```python
from build123d import *

# Parameters (mm, degrees)
SKETCH1_W                 = 5.2
SKETCH1_H                 = 14
SKETCH1_R                 = 3.2
SKETCH1_R_2               = 1.7
SKETCH1_R_3               = 2.75
BOSS_EXTRUDE1_DEPTH       = 10
SKETCH2_R                 = 2.6
CUT_EXTRUDE1_DEPTH        = 20
SKETCH3_R                 = 5.1
CUT_EXTRUDE2_DEPTH        = 15.2
BOSS_EXTRUDE2_DEPTH       = 0.45
BOSS_EXTRUDE2_DEPTH_BACK  = 0.45
SKETCH4_R                 = 5.1
SKETCH4_R_2               = 4.7
BOSS_EXTRUDE3_DEPTH       = 0.45
BOSS_EXTRUDE3_DEPTH_BACK  = 0.45
SKETCH5_R                 = 5.1
SKETCH5_R_2               = 4.7
CUT_EXTRUDE3_START        = -11
CUT_EXTRUDE3_OUTLINE_W    = 2.009975124
CUT_EXTRUDE3_OUTLINE_H    = 0.9
CUT_EXTRUDE3_OUTLINE_W_2  = 3
CUT_EXTRUDE3_OUTLINE_H_2  = 19.2
CUT_EXTRUDE3_DEPTH        = 12
SKETCH7_R                 = 12.5
CUT_EXTRUDE4_DEPTH        = 1
SKETCH8_R                 = 9.6
CUT_EXTRUDE5_DEPTH        = 1
SKETCH11_R                = 17
CUT_EXTRUDE6_DEPTH        = 6
BOSS_EXTRUDE4_OUTLINE_W   = 7.810507711
BOSS_EXTRUDE4_OUTLINE_H   = 8
BOSS_EXTRUDE4_OUTLINE_W_2 = 8
BOSS_EXTRUDE4_DEPTH       = 4.5
SKETCH13_R                = 2.125
CUT_EXTRUDE7_DEPTH        = 9.5
SKETCH16_W                = 0.189492289
SKETCH16_H                = 3.060913179
CUT_EXTRUDE8_DEPTH        = 4.5
FILLET1_R                 = 8
SKETCH19_R                = 12.5
CUT_EXTRUDE9_DEPTH        = 5
FILLET3_R                 = 3
CUT_EXTRUDE10_REACH       = 116.689
SKETCH20_R                = 1.7


with BuildPart() as part:
    # Sketch1 → Boss-Extrude1 (new body)
    with BuildSketch(Plane(origin=(0, 0, 0), x_dir=(0, 1, 0), z_dir=(0, 0, 1))):
        with BuildLine():
            Line((44.859200041, 91.5), (44.859200041, 77.3))
            Line((44.859200041, 77.3), (39.859200041, 77.3))
            Line((39.859200041, 77.3), (12.058048672, 27.485891377))
            ThreePointArc((12.058048672, 27.485891377), (12.182830244, 16.059150365), (22.1, 10.381499035))
            Line((22.1, 10.381499035), (33.6, 10.381499035))
            ThreePointArc((33.6, 10.381499035), (36.198905176, 18.091500699), (40.42011322, 25.047062246))
            Line((40.42011322, 25.047062246), (40.42011322, 39.489492289))
            Line((40.42011322, 39.489492289), (82.859200041, 39.489492289))
            Line((82.859200041, 39.489492289), (82.859200041, 77.3))
            Line((82.859200041, 77.3), (64.059200041, 77.3))
            Line((64.059200041, 77.3), (64.059200041, 91.5))
            Line((64.059200041, 91.5), (44.859200041, 91.5))
        make_face()
        with Locations((78.259200041, 52.489492289)):
            Rectangle(SKETCH1_W, SKETCH1_H, mode=Mode.SUBTRACT)
        with Locations(Location((22.1, 21.881499035, 0), (0, 0, 270))):
            Circle(SKETCH1_R, mode=Mode.SUBTRACT)
        with Locations(Location((65.859200041, 58.3, 0), (0, 0, 270))):
            Circle(SKETCH1_R_2, mode=Mode.SUBTRACT)
        with Locations(Location((56.359200041, 48.8, 0), (0, 0, 270))):
            Circle(SKETCH1_R_2, mode=Mode.SUBTRACT)
        with Locations(Location((46.859200041, 58.3, 0), (0, 0, 270))):
            Circle(SKETCH1_R_2, mode=Mode.SUBTRACT)
        with Locations(Location((56.359200041, 58.3, 0), (0, 0, 270))):
            Circle(SKETCH1_R_3, mode=Mode.SUBTRACT)
        with Locations(Location((56.359200041, 67.8, 0), (0, 0, 270))):
            Circle(SKETCH1_R_2, mode=Mode.SUBTRACT)
    extrude(amount=BOSS_EXTRUDE1_DEPTH)

    # Sketch2 → Cut-Extrude1 (cut)
    with BuildSketch(Plane.XZ.offset(-44.859200041)):
        with Locations(Location((-82.4, 5, 0), (0, 0, 270))):
            Circle(SKETCH2_R)
    extrude(amount=-CUT_EXTRUDE1_DEPTH, mode=Mode.SUBTRACT)

    # Sketch3 → Cut-Extrude2 (cut)
    with BuildSketch(Plane(origin=(0, 46.859200041, 0), x_dir=(-1, 0, 0), z_dir=(0, -1, 0))):
        with Locations((82.4, -5)):
            Circle(SKETCH3_R)
    extrude(amount=-CUT_EXTRUDE2_DEPTH, mode=Mode.SUBTRACT)

    # Sketch4 → Boss-Extrude2 (add, two sides: drawn at the far end of the back side and taken through both)
    with BuildSketch(Plane(origin=(0, 51.909200041, 0), x_dir=(-1, 0, 0), z_dir=(0, -1, 0)).offset(-BOSS_EXTRUDE2_DEPTH_BACK)):
        with Locations((82.4, -5)):
            Circle(SKETCH4_R)
        with Locations(Location((82.4, -5, 0), (0, 0, 90))):
            Circle(SKETCH4_R_2, mode=Mode.SUBTRACT)
    extrude(amount=BOSS_EXTRUDE2_DEPTH + BOSS_EXTRUDE2_DEPTH_BACK)

    # Sketch5 → Boss-Extrude3 (add, two sides: drawn at the far end of the back side and taken through both)
    with BuildSketch(Plane(origin=(0, 59.009200041, 0), x_dir=(1, 0, 0), z_dir=(0, 1, 0)).offset(-BOSS_EXTRUDE3_DEPTH_BACK)):
        with Locations((-82.4, -5)):
            Circle(SKETCH5_R)
        with Locations(Location((-82.4, -5, 0), (0, 0, 90))):
            Circle(SKETCH5_R_2, mode=Mode.SUBTRACT)
    extrude(amount=BOSS_EXTRUDE3_DEPTH + BOSS_EXTRUDE3_DEPTH_BACK)

    # Cut-Extrude3: read off the stored shape, not the designer's step
    # Cut-Extrude3 outline → Cut-Extrude3 (cut)
    with BuildSketch(Plane.XY.offset(10).offset(CUT_EXTRUDE3_START)):
        with Locations((-82.4, 59.009200041)):
            Rectangle(CUT_EXTRUDE3_OUTLINE_W, CUT_EXTRUDE3_OUTLINE_H)
        with Locations((-82.4, 51.909200041)):
            Rectangle(CUT_EXTRUDE3_OUTLINE_W, CUT_EXTRUDE3_OUTLINE_H)
        with Locations((-90, 54.459200041)):
            Rectangle(CUT_EXTRUDE3_OUTLINE_W_2, CUT_EXTRUDE3_OUTLINE_H_2)
    extrude(amount=CUT_EXTRUDE3_DEPTH, mode=Mode.SUBTRACT)

    # Sketch7 → Cut-Extrude4 (cut)
    with BuildSketch(Plane.XY.offset(10)):
        with Locations((-21.881499035, 22.1)):
            Circle(SKETCH7_R)
    extrude(amount=-CUT_EXTRUDE4_DEPTH, mode=Mode.SUBTRACT)

    # Sketch8 → Cut-Extrude5 (cut)
    with BuildSketch(Plane.XY.offset(9)):
        with Locations((-21.881499035, 22.1)):
            Circle(SKETCH8_R)
    extrude(amount=-CUT_EXTRUDE5_DEPTH, mode=Mode.SUBTRACT)

    # Sketch11 → Cut-Extrude6 (cut)
    with BuildSketch(Plane.XY.offset(10)):
        with Locations((-58.3, 56.359200041)):
            Circle(SKETCH11_R)
    extrude(amount=-CUT_EXTRUDE6_DEPTH, mode=Mode.SUBTRACT)

    # Boss-Extrude4: read off the stored shape, not the designer's step
    # Boss-Extrude4 outline → Boss-Extrude4 (add)
    with BuildSketch(Plane(origin=(0, 0, 0), x_dir=(1, 0, 0), z_dir=(0, 0, -1))):
        with Locations((-43.394746145, -71.359200041)):
            Rectangle(BOSS_EXTRUDE4_OUTLINE_W, BOSS_EXTRUDE4_OUTLINE_H)
        Polygon((-47.3, -45.359200041), (-39.489492289, -45.359200041), (-39.489492289, -40.42011322), (-39.3, -40.42011322), (-39.3, -37.359200041), (-47.3, -37.359200041), align=None)
        with Locations((-73.3, -71.359200041)):
            Rectangle(BOSS_EXTRUDE4_OUTLINE_W_2, BOSS_EXTRUDE4_OUTLINE_H)
        with Locations((-73.3, -41.359200041)):
            Rectangle(BOSS_EXTRUDE4_OUTLINE_W_2, BOSS_EXTRUDE4_OUTLINE_H)
    extrude(amount=BOSS_EXTRUDE4_DEPTH)

    # Sketch13 → Cut-Extrude7 (cut)
    with BuildSketch(Plane(origin=(0, 0, -4.5), x_dir=(1, 0, 0), z_dir=(0, 0, -1))):
        with Locations(Location((-43.3, -41.359200041, 0), (0, 0, 180))):
            Circle(SKETCH13_R)
        with Locations(Location((-43.3, -71.359200041, 0), (0, 0, 180))):
            Circle(SKETCH13_R)
        with Locations(Location((-73.3, -71.359200041, 0), (0, 0, 180))):
            Circle(SKETCH13_R)
        with Locations(Location((-73.3, -41.359200041, 0), (0, 0, 180))):
            Circle(SKETCH13_R)
    extrude(amount=-CUT_EXTRUDE7_DEPTH, mode=Mode.SUBTRACT)

    # Sketch16 → Cut-Extrude8 (cut)
    with BuildSketch(Plane(origin=(0, 0, -4.5), x_dir=(1, 0, 0), z_dir=(0, 0, -1))):
        with Locations((-39.394746145, -38.88965663)):
            Rectangle(SKETCH16_W, SKETCH16_H)
    extrude(amount=-CUT_EXTRUDE8_DEPTH, mode=Mode.SUBTRACT)

    # Fillet1
    # the kernel refuses this fillet: 8 mm, written as the material it adds along each edge
    with BuildSketch(Plane(origin=(-39.489492289, 40.42011322, 0), x_dir=(0, 1, 0), z_dir=(0, 0, 1))) as fillet1_piece_1:
        with BuildLine():
            CenterArc((FILLET1_R, -FILLET1_R), FILLET1_R, 90, 90)
            Line((0, -FILLET1_R), (0, 0))
            Line((0, 0), (FILLET1_R, 0))
        make_face()
    extrude(amount=10)
    # the kernel refuses this fillet: 8 mm, written as the material it takes off along each edge
    with BuildSketch(Plane(origin=(-25.047062246, 40.42011322, -6.434675881), x_dir=(-1, 0, 0), z_dir=(0, 0, 1))) as fillet1_2_piece_1:
        with BuildLine():
            CenterArc((2.573870352, 8), FILLET1_R, 236.049500449, 33.950499551)
            ThreePointArc((-1.893941258, 1.363836996), (-0.936214399, 0.696855523), (0, 0))
            Line((0, 0), (2.573870352, 0))
        make_face()
    extrude(amount=22.869351762, mode=Mode.SUBTRACT)
    with BuildSketch(Plane(origin=(-10.381499035, 33.6, -14.879687817), x_dir=(-0.9588293573098585, 0.2839828578642794, 0), z_dir=(0, 0, 1))) as fillet1_2_piece_2:
        with BuildLine():
            CenterArc((5.98040435, 7.978695466), FILLET1_R, 196.498058708, 69.319545905)
            Line((-1.690230508, 5.706832603), (0, 0))
            ThreePointArc((0, 0), (2.698475134, 0.098533472), (5.396950267, 0))
        make_face()
    extrude(amount=39.759375634, mode=Mode.SUBTRACT)

    # Sketch19 → Cut-Extrude9 (cut)
    with BuildSketch(Plane.XY.offset(10)):
        with Locations((-21.881499035, 22.1)):
            Circle(SKETCH19_R)
    extrude(amount=-CUT_EXTRUDE9_DEPTH, mode=Mode.SUBTRACT)

    # Fillet3
    # the kernel refuses this fillet: 3 mm, written as the material it takes off along each edge
    with BuildSketch(Plane(origin=(-10.381499035, 26.998979486, 14.214960222), x_dir=(9.684312598090364e-12, 1.0, -1.847411112972132e-14), z_dir=(0, 0, -1))) as fillet3_piece_1:
        with BuildLine():
            CenterArc((3.039490322, 1.812802001), FILLET3_R, 217.17613817, 22.016092035)
            ThreePointArc((1.503012295, -0.763869354), (0.76439954, -0.356565251), (0, 0))
            Line((0, 0), (0.649145388, 0))
        make_face()
    extrude(amount=9.214960222, mode=Mode.SUBTRACT)
    with BuildSketch(Plane(origin=(-31.763744729, 14.445509812, 5), x_dir=(-0.35715309500497466, 0.9340458590071301, -7.501643631045315e-14), z_dir=(0, 0, 1))) as fillet3_piece_2:
        with BuildLine():
            CenterArc((8.109181309, 2.871430927), FILLET3_R, 129.90874339, 123.256431286)
            Line((6.184481226, 5.172632698), (0, 0))
            ThreePointArc((0, 0), (3.620170227, 0.53570447), (7.240340454, 0))
        make_face()
    extrude(amount=25.156254778, mode=Mode.SUBTRACT)

    # Sketch20 → Cut-Extrude10 (cut, up to next)
    with BuildSketch(Plane(origin=(0, 82.859200041, 0), x_dir=(-1, 0, 0), z_dir=(0, 1, 0)), mode=Mode.PRIVATE) as cut_extrude10_sk1:
        with Locations(Location((52.489492289, 5, 0), (0, 0, 90))):
            Circle(SKETCH20_R)
    cut_extrude10_tool1 = extrude(cut_extrude10_sk1.sketch, amount=-CUT_EXTRUDE10_REACH, mode=Mode.PRIVATE) & part.part
    add(cut_extrude10_tool1.solids().sort_by_distance((-52.489492, 82.8592, 5))[0], mode=Mode.SUBTRACT)


solid = part.part
```
CAD build for the part. Positions are in the model's coordinates, mm. A direction names the side the tool comes from. Round coordinates to 2 decimals unless told otherwise and drop trailing zeros. Write each loop counter-clockwise with the first axis right and the second up, starting at its lowest first coordinate (ties: lowest second). Pieces come first, ordered by that corner, then holes. Notation, with made-up numbers: M 31.25,-14.5 L 36.25,-14.5 A19 ccw 36.25,1.5 Z; hole C 7.25,74.25 d1. An arc over 180 degrees is marked long. One line per question, with ' | ' between items.
1. Pin check, flat tips, straight feed: pin 1 Ø5 at (x, z) = (-74, -2) entering from -Y; pin 2 Ø4 at (y, z) = (48.5, 7) entering from +X; pin 3 Ø3.5 at (x, z) = (-44.5, -2.5) entering from -Y. Stop position of each tip, or through.
Working result:
pin 1: y = 37.18 | pin 2: x = -39.26 | pin 3: y = 37.36
2. Cut at A-A on x = -58.3. Write the cut outline in (y, z).
Working result:
outline: M 29.26,0 L 45.16,0 L 45.16,4 L 39.36,4 L 39.36,10 L 29.26,10 Z; M 48.56,0 L 53.61,0 L 53.61,4 L 48.56,4 Z; M 59.11,0 L 64.16,0 L 64.16,4 L 59.11,4 Z; M 67.56,0 L 75.66,0 L 75.66,10 L 73.36,10 L 73.36,4 L 67.56,4 Z; M 80.86,0 L 82.86,0 L 82.86,10 L 80.86,10 Z
3. Mould opens along Z. For faces 1 (the flat face through (-71.6, 73.1, -4.5)), 2 (the cylindrical face through (-71.61, 40.07, 0.18)), 3 (the cylindrical face through (-87.1, 51.9, 5.1)) say: pulls with the +Z half, pulls with the -Z half, needs draft (parallel to the pull), parting line crosses it, or undercut.
Working result:
face 1: pulls with the -Z half | face 2: needs draft | face 3: undercut
4. Probe L1, parallel to Y at x = -73.3, z = -0.5; L2, parallel to X at y = 49, z = 8.75; L3, parallel to X at y = 45.5, z = 5. List the from-to ranges inside material, lowest first. Write a range as from..to.
Working result:
L1: 37.36..39.23, 43.48..45.36, 67.36..69.23, 73.48..75.36 | L2: -88.5..-85.86, -78.94..-73.62, -42.98..-39.49 | L3: -88.5..-85, -79.8..-71.38, -45.22..-38.94
5. Cut at D-D on x = -68. Write the cut outline in (y, z), and give its area (3 significant figures).
Working result:
outline: M 34.67,0 L 54.67,0 L 54.67,4 L 42.4,4 L 42.4,10 L 34.67,10 Z; M 58.05,0 L 82.86,0 L 82.86,10 L 70.32,10 L 70.32,4 L 58.05,4 Z | area: 301 mm2
6. Which spindle directions (+Z, -Z, +X, -X, +Y, -Y) get a long thin tool onto all of the face, cutting with end or side? Do faces 4 (the cylindrical face through (-77.3, 49.1, 4.9)), 5 (the flat face through (-43, 41, 5)), 6 (the flat face through (-39.489, 66, 4)). Say none if no direction does.
Working result:
face 4: none | face 5: -Z | face 6: +Z, -Z, +X, +Y
7. Cut at B-B on z = -2. Count the separate pieces of the cut face and the enclosed holes in it, and give its area (3 significant figures).
Working result:
separate pieces: 4 | enclosed holes: 4 | area: 196 mm2
8. Cut at C-C on x = -82.4. Write the cut outline in (y, z).
Working result:
outline: M 44.86,0 L 46.86,0 L 46.86,2.4 L 44.86,2.4 Z; M 44.86,7.6 L 46.86,7.6 L 46.86,10 L 44.86,10 Z; M 62.06,0 L 64.06,0 L 64.06,2.4 L 62.06,2.4 Z; M 62.06,7.6 L 64.06,7.6 L 64.06,10 L 62.06,10 Z
